from build123d import *

# Parameters (mm, degrees)
F1_DEPTH = 225
F3_DEPTH = 100


with BuildPart() as f1:
    # F0 (on Top) → F1 (new body)
    with BuildSketch(Plane.XY):
        with BuildLine():
            Line((35, 50), (-35, 50))
            ThreePointArc((-35, 50), (-45.606602, 45.606602), (-50, 35))
            Line((-50, 35), (-50, -35))
            ThreePointArc((-50, -35), (-45.606602, -45.606602), (-35, -50))
            Line((-35, -50), (35, -50))
            ThreePointArc((35, -50), (45.606602, -45.606602), (50, -35))
            Line((50, -35), (50, 35))
            ThreePointArc((50, 35), (45.606602, 45.606602), (35, 50))
        make_face()
        with BuildLine():
            ThreePointArc((-40, 30), (-37.071068, 37.071068), (-30, 40))
            Line((-30, 40), (30, 40))
            ThreePointArc((30, 40), (37.071068, 37.071068), (40, 30))
            Line((40, 30), (40, -30))
            ThreePointArc((40, -30), (37.071068, -37.071068), (30, -40))
            Line((30, -40), (-30, -40))
            ThreePointArc((-30, -40), (-37.071068, -37.071068), (-40, -30))
            Line((-40, -30), (-40, 30))
        make_face(mode=Mode.SUBTRACT)
    extrude(amount=F1_DEPTH)

    # F2 (on face) → F3 (cut)
    with BuildSketch(Plane.YZ.offset(50)):
        Polygon((-50, 225), (-50, 167.264973), (50, 225), align=None)
        Polygon((50, 71.424828), (-50, 13.689801), (-50, 0), (50, 0), align=None)
    extrude(amount=-F3_DEPTH, mode=Mode.SUBTRACT)


solid = f1.part
Part model, mm, in its own coordinate system. A direction names the side the tool comes from. Coordinates: 2 decimals unless noted, no trailing zeros. Order: outer loops, then holes, each group sorted by start corner. A loop starts at its lowest first (then second) coordinate and runs counter-clockwise, first axis right, second up. Notation, with made-up numbers: M 26.25,-23.75 L 83.25,-23.75 A22 cw 83.25,-13.75 Z; hole C 45.25,-17 d3. An arc over 180 degrees is marked long. One line per question, with ' | ' between items.
Q1. Slice it at B-B (x = -6.5). Give the cut face in (y, z).
A:
outline: M -50,13.69 L -40,19.46 L -40,173.04 L -50,167.26 Z; M 40,65.65 L 50,71.42 L 50,225 L 40,219.23 Z
Q2. Two-plate mould, pull along X, no slides. Class faces 1 (the face through (40, 0, 118)), 2 (the face through (-45.72, -45.49, 93.67)), 3 (the face through (45.49, -45.72, 93.67)): +X half, -X half, draft (parallel to the pull), parting line (faces both ways), or undercut.
A:
face 1: undercut | face 2: -X half | face 3: +X half
Q3. Slice it at A-A (z = 88.5). Give the cut face in (x, y), and give its area (3 significant figures).
A:
outline: M -50,-35 A15 ccw -35,-50 L 35,-50 A15 ccw 50,-35 L 50,35 A15 ccw 35,50 L -35,50 A15 ccw -50,35 Z; hole M -40,-30 A10 ccw -30,-40 L 30,-40 A10 ccw 40,-30 L 40,30 A10 ccw 30,40 L -30,40 A10 ccw -40,30 Z | area: 3,490 mm^2
Q4. Pin check, flat tip, straight feed: P1, Ø5, axis at x = -28.5, z = 54.5, coming from the +Y side. Stop position of the tip, or through.
A:
P1: stops at y = -39.95
Q5. Slice it at D-D (z = 37). Give the cut face in (x, y), and give its area (3 significant figures).
A:
outline: M -50,-35 A15 ccw -35,-50 L 35,-50 A15 ccw 50,-35 L 50,-9.63 L 40,-9.63 L 40,-30 A10 cw 30,-40 L -30,-40 A10 cw -40,-30 L -40,-9.63 L -50,-9.63 Z | area: 1,550 mm^2
Q6. Slice it at C-C (y = -7). Give the cut face in (x, z).
A:
outline: M -50,38.52 L -40,38.52 L -40,192.09 L -50,192.09 Z; M 40,38.52 L 50,38.52 L 50,192.09 L 40,192.09 Z
Q7. 3-axis set-ups, long thin cutter, end or side, ignore diameter. For faces 4 (the face through (0, -40, 95)), 5 (the face through (50, 0, 118)): which of +Z, -Z, +X, -X, +Y, -Y reach the whole face in a straight line?
A:
face 4: +Z, -Z | face 5: +Z, -Z, +X, +Y, -Y
Q8. Drill centre lines: line 1 (Y direction, x = 10.5, z = 156); line 2 (X direction, y = 38, z = 140.5). Where is each one in solid material? Low to high.
A:
line 1: y = -50 to -40, 40 to 50 | line 2: x = -49.7 to -36, 36 to 49.7
